Input: part model. Units: mm. Frame: model coordinates. Round coordinates to 2 decimals unless told otherwise and drop trailing zeros. Loops run counter-clockwise (first coordinate to the right, second up) from the corner with the lowest first, then second, coordinate; pieces in that order, holes last.
1) Ray query, line 1 along X through (y, z) = (1.05, 0); line 2 along Z through (x, y) = (-129.9, 2.85) (3 decimals); line 3 along Z through (x, y) = (-123.9, 3.2) (3 decimals). Return the intervals inside material, ascending.
2) Section B-B, the plane x = 21. Return loops of the section in (y, z) (3 decimals), and give its area (3 significant figures).
3) First-contact query: pin 1 (1.4 mm diameter, centred on x = 3.5, y = 2, fed in from +Z) (3 decimals); pin 2 (2.5 mm diameter, centred on x = -124.5, y = 3, fed in from -Z) (3 decimals); pin 3 (1.4 mm diameter, centred on y = 1.5, z = 100.5, fed in from -X). Flat tips, straight axial feed; report the tip coordinate or a pass-through.
4) Section A-A, the plane y = 2.65. Return loops of the section in (x, z) (3 decimals), and give its area (3 significant figures).
from build123d import *

# Parameters (mm, degrees)
EXTRUDE_1_DEPTH     = 4.75
SKETCH_3_R          = 1.75
CUT_EXTRUDE_1_DEPTH = 4.75
SKETCH_4_R          = 2.15
CUT_EXTRUDE_2_DEPTH = 4.75


with BuildPart() as part:
    # 草圖1 → 填料-伸長1 (new body)
    with BuildSketch(Plane(origin=(0, 0, 0), x_dir=(1, 0, 0), z_dir=(0, 1, 0))):
        Polygon((-105.4, 97.625), (-150.4, 97.625), (-150.4, -97.625), (-105.4, -97.625), (-105.4, -102.375), (-25.4, -102.375), (-25.4, -97.625), (25.4, -97.625), (25.4, -102.375), (105.4, -102.375), (105.4, -97.625), (105.4, 97.625), (105.4, 102.375), (25.4, 102.375), (25.4, 97.625), (-25.4, 97.625), (-25.4, 102.375), (-105.4, 102.375), align=None)
    extrude(amount=EXTRUDE_1_DEPTH)

    # 草圖3 → 除料-伸長1 (cut)
    with BuildSketch(Plane(origin=(0, 4.75, 0), x_dir=(1, 0, 0), z_dir=(0, 1, 0))):
        with Locations(Location((-123.9, 0, 0), (0, 0, 270))):
            Circle(SKETCH_3_R)
        with Locations(Location((-142.9, 0, 0), (0, 0, 270))):
            Circle(SKETCH_3_R)
    extrude(amount=-CUT_EXTRUDE_1_DEPTH, mode=Mode.SUBTRACT)

    # 草圖4 → 除料-伸長2 (cut)
    with BuildSketch(Plane(origin=(0, 4.75, 0), x_dir=(1, 0, 0), z_dir=(0, 1, 0))):
        with Locations(Location((-105.4, -89.725, 0), (0, 0, 270))):
            Circle(SKETCH_4_R)
        with Locations(Location((-129.9, -89.725, 0), (0, 0, 270))):
            Circle(SKETCH_4_R)
        with Locations(Location((-105.4, 89.725, 0), (0, 0, 270))):
            Circle(SKETCH_4_R)
        with Locations(Location((-129.9, 89.725, 0), (0, 0, 270))):
            Circle(SKETCH_4_R)
    extrude(amount=-CUT_EXTRUDE_2_DEPTH, mode=Mode.SUBTRACT)


solid = part.part
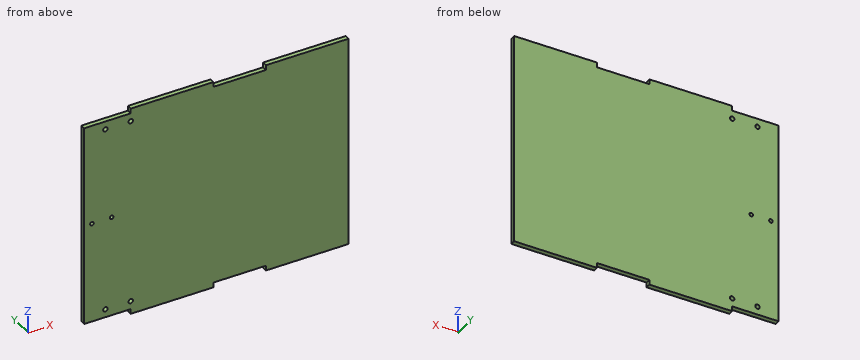
Final values:
1. line 1: x = -150.4 to -144.65, -141.15 to -125.65, -122.15 to 105.4
1. line 2: z = -97.625 to -91.875, -87.575 to 87.575, 91.875 to 97.625
1. line 3: z = -97.625 to -1.75, 1.75 to 97.625
2. outline: (0, -97.625) - (4.75, -97.625) - (4.75, 97.625) - (0, 97.625) - close
2. area: 927 mm2
3. pin 1: stops at z = 97.625
3. pin 2: stops at z = -97.625
3. pin 3: stops at x = -105.4
4. outline: (-150.4, -97.625) - (-105.4, -97.625) - (-105.4, -102.375) - (-25.4, -102.375) - (-25.4, -97.625) - (25.4, -97.625) - (25.4, -102.375) - (105.4, -102.375) - (105.4, 102.375) - (25.4, 102.375) - (25.4, 97.625) - (-25.4, 97.625) - (-25.4, 102.375) - (-105.4, 102.375) - (-105.4, 97.625) - (-150.4, 97.625) - close; hole circle Ø3.5 at (-142.9, 0); hole circle Ø4.3 at (-129.9, -89.725); hole circle Ø4.3 at (-129.9, 89.725); hole circle Ø3.5 at (-123.9, 0); hole circle Ø4.3 at (-105.4, -89.725); hole circle Ø4.3 at (-105.4, 89.725)
4. area: 51,400 mm2
